Design review of the part built by this model. Coordinates are the model's own, in mm. Face numbers are marked on the shaded views. A direction names the side the tool comes from. Coordinates: 2 decimals unless noted, no trailing zeros. Write each loop counter-clockwise with the first axis right and the second up, starting at its lowest first coordinate (ties: lowest second). Pieces come first, ordered by that corner, then holes.
Q1. Take a section at A-A (y = 0). Give the boundary of the cut face in (x, z).
Q2. Take a section at C-C (x = 6.25). Give the boundary of the cut face in (y, z), and give its area (3 significant figures).
Q3. Insertion check: pin 1 (2 mm diameter, centred on x = 4.5, z = -20, fed in from -Y); pin 2 (4.5 mm diameter, centred on x = 2, y = -32, fed in from -Z); pin 3 (5 mm diameter, centred on x = 10, z = -22, fed in from -Y). Each pin has a flat end and moves straight along its axis. Give the tip position at first contact, or say it passes through.
Q4. For probe 1 along Z at (x, y) = (7.5, 0); probe 2 along Z at (x, y) = (1, -4.5); probe 3 along Y at (x, z) = (1.25, -0.5), list the stretches that pass through material, from the lowest coordinate up.
Q5. Mouldability with a two-part tool opening along Y and no side actions: class the marked faces 1, 2 and 3 as pulls with the +Y half, pulls with the -Y half, needs draft (parallel to the pull), parting line crosses it, or undercut.
Q6. Machinability: for the marked faces 4 and 5, which of the approach directions +Z, -Z, +X, -X, +Y, -Y give a long, thin tool a straight path to every point of the face, cutting with its end or side? Answer none if there is none.
Q7. Take a section at B-B (x = 2.25). Give the boundary of the cut face in (y, z), and give its area (3 significant figures).
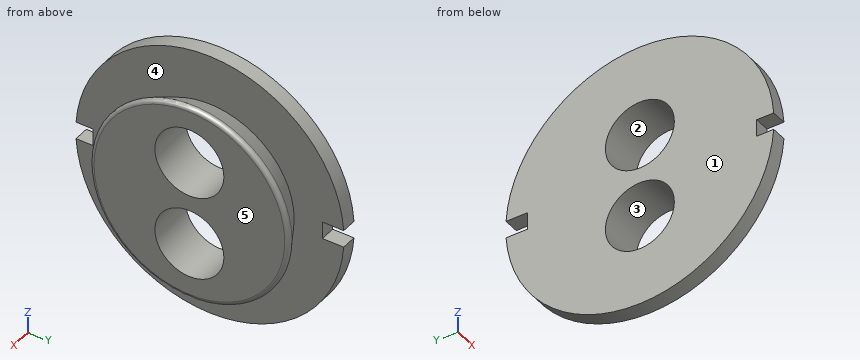
Autodesk Inventor part; units mm, degrees
ref_plane "YZ Plane" through (0, 0, 0) normal (1, 0, 0) x (0, 1, 0)
ref_plane "XZ Plane" through (0, 0, 0) normal (0, 1, 0) x (-1, 0, 0)
ref_plane "XY Plane" through (0, 0, 0) normal (0, 0, 1) x (1, 0, 0)
sketch "Эскиз1" plane through (0, 0, 0) normal (0, 0, 1) x (1, 0, 0)
  line L0 (0, 0) -> (4, 0)
  line L1 (4, 0) -> (4, -35)
  line L2 (4, -35) -> (0, -35)
  line L3 (0, -35) -> (0, 0)
  line L4 (4, 0) -> (12, 0)
  line L5 (12, 0) -> (12, -24.8868)
  line L6 (12, -26.6188) -> (4, -26.6188)
  line L7 (4, -26.6188) -> (4, 0)
  line L8 (4, 0) -> (4, -22)
  line L9 (4, -22) -> (10.5, -25.7528)
  arc A0 (10.5, -25.7528) -> (12, -24.8868) centre (11, -24.8868) ccw
  dimension "d0" = 4
  dimension "d1" = 35
  dimension "d2" = 8
  dimension "d4" = 22
  dimension "d36" = 60
  dimension "d37" = 1
revolve "Вращение1" add sketch "Эскиз1" angle 360 about axis through (0, 0, 0) along (1, 0, 0)
mirror "Зеркальное отражение1" [suppressed]
sketch "Эскиз2" plane through (12, 0, 0) normal (1, 0, 0) x (0, 0, -1)
  circle A0 centre (11, 0) radius 9
  circle A1 centre (-11, 0) radius 9
  point P0 (0, 0)
  dimension "d6" = 18
  dimension "d7" = 18
  dimension "d8" = 11
  dimension "d9" = 11
  dimension "d10" = 40
hole "Отверстие1" at (12, 0, 11) direction (-1, 0, 0) diameter 18 end through all
hole "Отверстие2" at (12, 0, -11) direction (-1, 0, 0) diameter 18 end through all
sketch "Эскиз3" plane through (4, 0, 0) normal (1, 0, 0) x (0, 0, -1)
  line L0 (-2.25, 35) -> (2.25, 35)
  line L1 (2.25, 35) -> (2.25, 29.3705)
  line L2 (2.25, 29.3705) -> (-2.25, 29.3705)
  line L3 (-2.25, 29.3705) -> (-2.25, 35)
  circle A0 centre (0, 0) radius 35
  line L4 (0, 35) -> (0, 30.5)
  line L5 (0, -35) -> (0, -30.5)
  line L6 (-2.25, -30.5) -> (2.25, -30.5)
  line L7 (2.25, -30.5) -> (2.25, -35)
  line L8 (2.25, -35) -> (-2.25, -35)
  line L9 (-2.25, -35) -> (-2.25, -30.5)
  point P0 (0, 0)
  dimension "d25" = 4.5
  dimension "d26" = 4.5
  dimension "d27" = 2.25
  dimension "d28" = 0
  dimension "d29" = 4.5
  dimension "d30" = 4.5
  dimension "d31" = 4.5
  dimension "d32" = 2.25
  dimension "d33" = 0
extrude "Выдавливание1" cut sketch "Эскиз3" against normal blind 4 contours L0 A0 L3 | L0 L1 A0 | A0 L1 L2 L3 | L9 L6 L5 A0 | A0 L8 L9 | L5 L6 L7 A0 | A0 L7 L8
equation "\"d0\" = 0.5 * hFlange"
equation "\"d1\" = 0.5 * dOuter"
equation "\"d2\" = hMount"
equation "\"d4\" = 0.5 * dMinimal"
equation "\"d36\" = angleMount"
equation "\"d6\" = dHoles"
equation "\"d7\" = dHoles"
equation "\"d11\" = dHoles"
equation "\"d18\" = dHoles"
equation "\"d25\" = wSlot"
equation "\"d26\" = hSlot"
equation "\"d27\" = 0.5 * wSlot"
equation "\"d29\" = hSlot"
equation "\"d30\" = hSlot"
equation "\"d31\" = wSlot"
equation "\"d32\" = 0.5 * wSlot"
equation "\"hFlange\" = 8"
equation "\"dMinimal\" = 44"
equation "\"angleMount\" = 60deg"
equation "\"dHoles\" = 18"
equation "\"r2holes\" = 11"
equation "\"hMount\" = 8"
equation "\"wSlot\" = 4.5"
equation "\"hSlot\" = 4.5"
properties part number "SpacerCorrect"
Response:
1. outline: (0, -35) - (4, -35) - (4, -22) - (10.5, -25.75) arc R1 ccw to (12, -24.89) - (12, -20) - (0, -20) - close; (0, -2) - (12, -2) - (12, 2) - (0, 2) - close; (0, 20) - (12, 20) - (12, 24.89) arc R1 ccw to (10.5, 25.75) - (4, 22) - (4, 35) - (0, 35) - close
2. outline: circle Ø46.6 at (0, 0); hole circle Ø18 at (0, -11); hole circle Ø18 at (0, 11)
2. area: 1,200 mm2
3. pin 1: stops at y = -29.31
3. pin 2: stops at z = -18.44
3. pin 3: stops at y = -16.84
4. probe 1: z = -24.02 to -20, -2 to 2, 20 to 24.02
4. probe 2: z = -34.71 to -18.79, -3.21 to 3.21, 18.79 to 34.71
4. probe 3: y = -30.5 to 29.37
5. face 1: needs draft
5. face 2: undercut
5. face 3: undercut
6. face 4: none
6. face 5: +Z, -Z, +X, +Y, -Y
7. outline: (-34.93, -2.25) arc R35 ccw to (34.93, -2.25) - (29.37, -2.25) - (29.37, 2.25) - (34.93, 2.25) arc R35 ccw to (-34.93, 2.25) - (-30.5, 2.25) - (-30.5, -2.25) - close; hole circle Ø18 at (0, -11); hole circle Ø18 at (0, 11)
7. area: 3,290 mm2
